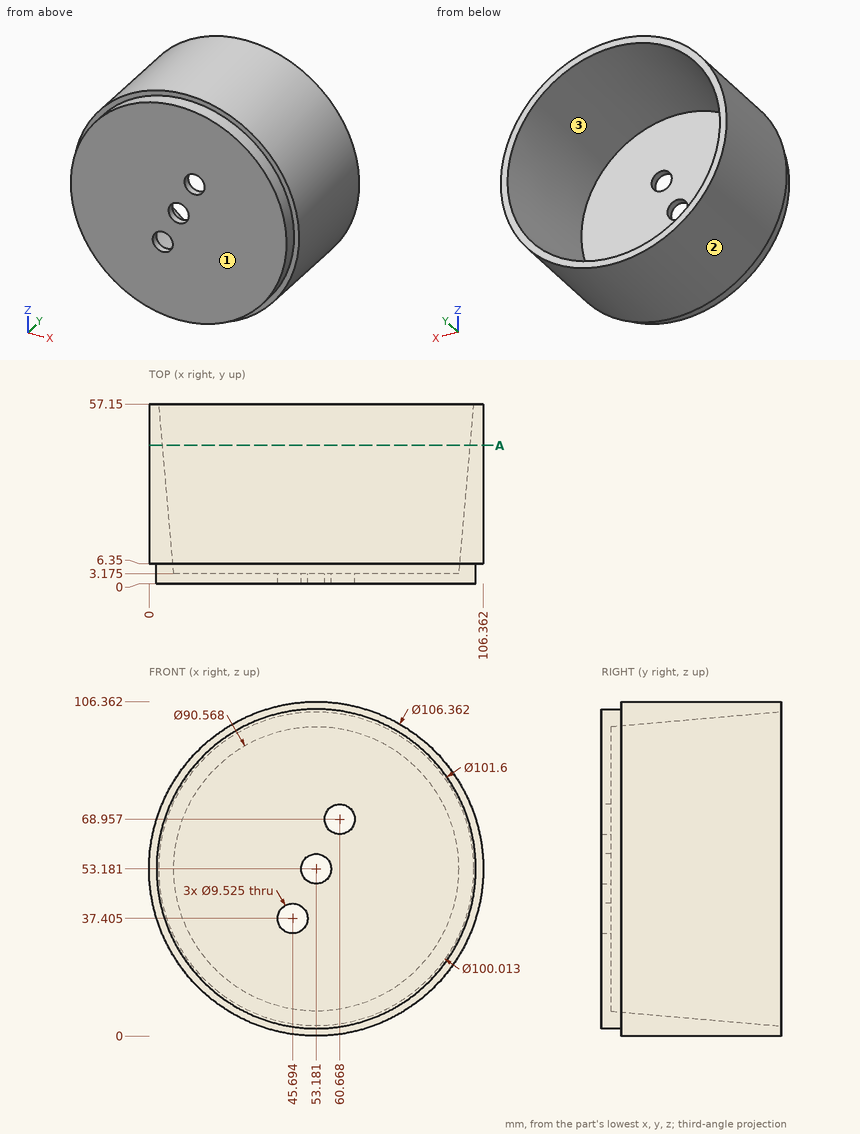
Drawing for the job (mm, zero at the part's lowest x, y, z). Coordinates: 2 decimals unless noted, no trailing zeros. Order: outer loops, then holes, each group sorted by start corner. A loop starts at its lowest first (then second) coordinate and runs counter-clockwise, first axis right, second up. Notation, with made-up numbers: (23, 27) -> (68, 27) arc R27 cw to (68, 47) -> close; hole circle Ø3 at (-18.75, 31.25). An arc over 180 degrees is marked (long way). Return JSON: item names as keys, results as strings.
Item 1: Wall check: line 1 along Y through (x, z) = (70, 66) (1 decimal); line 2 along X through (y, z) = (52, 39.5); line 3 along X through (y, z) = (28.5, 28) (1 decimal). Give the ranges that are in metal, low to high. Write a range as from..to.
Model answer:
{"line 1": "y = 0..3.2", "line 2": "x = 1.79..5.55, 100.81..104.57", "line 3": "x = 6.3..12.9, 93.5..100"}
Item 2: Pin check, flat tips, straight feed: P1, Ø8, axis at y = 38.5, z = 15, coming from the +X side; P2, Ø4, axis at x = 71, y = 12.5, coming from the -Z side; P3, Ø12, axis at x = 88, y = 8.5, coming from the +Z side. Stop position of each tip, or through.
Model answer:
{"P1": "stops at x = 93.92", "P2": "stops at z = 2.41", "P3": "stops at z = 97.88"}
Item 3: Slice it at A-A (y = 44). Write the cut outline in (x, z) (1 decimal), then the cut area to 3 significant figures.
Model answer:
{"outline": "circle Ø106.4 at (53.2, 53.2); hole circle Ø97.7 at (53.2, 53.2)", "area": "1,390 mm²"}
Item 4: Mould opens along Z. For the marked faces 1, 2 and 3 say: pulls with the +Z half, pulls with the -Z half, needs draft (parallel to the pull), parting line crosses it, or undercut.
Model answer:
{"face 1": "needs draft", "face 2": "parting line crosses it", "face 3": "undercut"}
